from build123d import *

# Parameters (mm, degrees)
SALIENTE_EXTRUIR1_DEPTH = 21
REDONDEO1_R             = 10.5
CROQUIS2_R              = 16
SALIENTE_EXTRUIR2_DEPTH = 38
CROQUIS3_R              = 10
CORTAR_EXTRUIR1_DEPTH   = 74
CROQUIS4_R              = 3
CORTAR_EXTRUIR2_DEPTH   = 25
MATRIZC1_COUNT          = 3


with BuildPart() as part:
    # Croquis1 → Saliente-Extruir1 (new body)
    with BuildSketch(Plane.XY):
        with BuildLine():
            Line((15, 20.207259422), (33.97114317, 31.160254038))
            Line((33.97114317, 31.160254038), (43.97114317, 13.839745962))
            Line((43.97114317, 13.839745962), (25, 2.886751346))
            ThreePointArc((25, 2.886751346), (14.019237886, -8.094010768), (10, -23.094010768))
            Line((10, -23.094010768), (10, -45))
            Line((10, -45), (-10, -45))
            Line((-10, -45), (-10, -23.094010768))
            ThreePointArc((-10, -23.094010768), (-14.019237886, -8.094010768), (-25, 2.886751346))
            Line((-25, 2.886751346), (-43.97114317, 13.839745962))
            Line((-43.97114317, 13.839745962), (-33.97114317, 31.160254038))
            Line((-33.97114317, 31.160254038), (-15, 20.207259422))
            ThreePointArc((-15, 20.207259422), (0, 16.188021535), (15, 20.207259422))
        make_face()
    extrude(amount=SALIENTE_EXTRUIR1_DEPTH)

    # Redondeo1
    redondeo1_edges = [part.edges().sort_by_distance(p)[0] for p in [
        (38.97114317, 22.5, 21),
        (-38.97114317, 22.5, 21),
        (0, -45, 21),
    ]]
    fillet(redondeo1_edges, radius=REDONDEO1_R)

    # Croquis2 → Saliente-Extruir2 (add)
    with BuildSketch(Plane.XY.offset(21)):
        with Locations(Location((0, 0, 0), (0, 0, 180))):
            Circle(CROQUIS2_R)
    extrude(amount=SALIENTE_EXTRUIR2_DEPTH)

    # Croquis3 → Cortar-Extruir1 (cut)
    with BuildSketch(Plane.XY.offset(59)):
        Circle(CROQUIS3_R)
    extrude(amount=-CORTAR_EXTRUIR1_DEPTH, mode=Mode.SUBTRACT)

    # Croquis4 → Cortar-Extruir2 (cut)
    with BuildSketch(Plane(origin=(5, 8.660254038, 0), x_dir=(0.866025403784439, -0.4999999999999993, 0), z_dir=(0.4999999999999993, 0.866025403784439, 0))):
        with Locations(Location((-34.5, -10.5, 0), (0, 0, 180))):
            Circle(CROQUIS4_R)
    cortar_extruir2 = extrude(amount=-CORTAR_EXTRUIR2_DEPTH, mode=Mode.SUBTRACT)

    # MatrizC1: Cortar-Extruir2 ×3 about axis
    matrizc1_axis = Axis((0, 0, 59), (0, 0, -1))
    for i in range(1, MATRIZC1_COUNT):
        add(cortar_extruir2.rotate(matrizc1_axis, i * 360 / MATRIZC1_COUNT), mode=Mode.SUBTRACT)


solid = part.part
Design review of the part built by this model. Coordinates are the model's own, in mm. A direction names the side the tool comes from. Round coordinates to 2 decimals unless told otherwise and drop trailing zeros. Write each loop counter-clockwise with the first axis right and the second up, starting at its lowest first coordinate (ties: lowest second). Pieces come first, ordered by that corner, then holes.
Item 1: Consider section C-C on z = 15. Give the boundary of the cut face in (x, y).
Item 2: Consider section B-B on y = -33. Give the boundary of the cut face in (x, z), and give its area (3 significant figures).
Item 3: Wall thickness on L1, parallel to Y at x = -4, z = 10; L2, parallel to Y at x = 0, z = 39.5; L3, parallel to Z at x = 6.5, y = -16: over which ranges is each line inside the solid? List them lowest first.
Item 4: For pin 1 Ø1 at (y, z) = (-7.5, 25.5) entering from +X; pin 2 Ø12 at (x, z) = (-1, 8.5) entering from +Y; pin 3 Ø5 at (y, z) = (-16, 44) entering from -X; pin 4 Ø5 at (y, z) = (-34.5, 10.5) entering from -X, all flat-tipped, find the tip position at first contact; note any pin that passes through.
Item 5: Consider section D-D on y = 12. Count the separate pieces of the cut face and the enclosed holes in it, and give its area (3 significant figures).
Item 6: For faces 4 (the flat face through (22.245, 24.39, 8.02)), 5 (the flat face through (10, -31, 10)), 6 (the flat face through (-10, -32, 8)), 7 (the cylindrical face through (3.47, 15.62, 39.73)), list the 3-axis set-ups (+Z, -Z, +X, -X, +Y, -Y) from which the entire face can be reached by the end or side of a thin tool; tool diameter is ignored.
Item 7: Draft analysis for pull direction Z (two halves, no side actions). For faces 1 (the flat face through (-10.4, -0.2, 59)), 2 (the flat face through (-39.04, 22.38, 5.18)), 3 (the cylindrical face through (27.352, 15.63, 10.632)), state which applies: released by +Z, released by -Z, zero draft, split by the parting line, or undercut.
Item 8: Consider section A-A on x = 0. Give the boundary of the cut face in (y, z).
Check values:
1. outline: (-43.09, 13.33) - (-25, 2.89) arc R30 cw to (-10, -23.09) - (-10, -43.99) - (10, -43.99) - (10, -23.09) arc R30 cw to (25, 2.89) - (43.09, 13.33) - (33.09, 30.65) - (15, 20.21) arc R30 cw to (-15, 20.21) - (-33.09, 30.65) - close; hole circle Ø20 at (0, 0)
2. outline: (-10, 0) - (10, 0) - (10, 7.9) - (-10, 7.9) - close; (-10, 13.1) - (10, 13.1) - (10, 21) - (-10, 21) - close
2. area: 316 mm2
3. L1: y = -45 to -37.46, -31.54 to -9.17, 9.17 to 16.46
3. L2: y = -16 to -10, 10 to 16
3. L3: z = 0 to 21
4. pin 1: stops at x = 14.39
4. pin 2: stops at y = 17.02
4. pin 3: stops at x = -8.59
4. pin 4: passes through
5. separate pieces: 1
5. enclosed holes: 2
5. area: 2,440 mm2
6. face 4: +Z, -Z, +Y
6. face 5: +Z, -Z, +X, -Y
6. face 6: +Z, -Z, -X, -Y
6. face 7: +Z
7. face 1: released by +Z
7. face 2: zero draft
7. face 3: undercut
8. outline: (-45, 0) - (-10, 0) - (-10, 59) - (-16, 59) - (-16, 21) - (-34.5, 21) arc R10.5 ccw to (-45, 10.5) - close; (10, 0) - (16.19, 0) - (16.19, 21) - (16, 21) - (16, 59) - (10, 59) - close; hole circle Ø6 at (-34.5, 10.5)
